from build123d import *

# Parameters (mm, degrees)
BOSS_EXTRUDE1_DEPTH     = 7.62
SKETCH2_W               = 85.677392152
SKETCH2_H               = 16.256
CUT_EXTRUDE1_DEPTH      = 1
CUT_EXTRUDE1_DEPTH_BACK = 8.62
FILLET1_R               = 5.08
SKETCH3_W               = 10.16
SKETCH3_H               = 7.62
CUT_EXTRUDE2_DEPTH      = 8.62
SKETCH4_W               = 25.4
SKETCH4_H               = 10.16
CUT_EXTRUDE3_DEPTH      = 8.62


with BuildPart() as part:
    # Sketch1 → Boss-Extrude1 (new body)
    with BuildSketch(Plane(origin=(0, 0, 0), x_dir=(1, 0, 0), z_dir=(0, 1, 0))):
        with BuildLine():
            Line((-88.9, 0), (-88.9, 76.2))
            ThreePointArc((-88.9, 76.2), (0, 165.1), (88.9, 76.2))
            Line((88.9, 76.2), (88.9, 0))
            ThreePointArc((88.9, 0), (0, -88.9), (-88.9, 0))
        make_face()
    extrude(amount=BOSS_EXTRUDE1_DEPTH)

    # Sketch2 → Cut-Extrude1 (cut, two sides)
    with BuildSketch(Plane(origin=(0, 7.62, 0), x_dir=(1, 0, 0), z_dir=(0, 1, 0))) as cut_extrude1_sk:
        with Locations((0, -58.235236409)):
            Rectangle(SKETCH2_W, SKETCH2_H)
        with Locations((0, 134.435236409)):
            Rectangle(SKETCH2_W, SKETCH2_H)
    extrude(amount=CUT_EXTRUDE1_DEPTH, mode=Mode.SUBTRACT)
    extrude(cut_extrude1_sk.sketch, amount=-CUT_EXTRUDE1_DEPTH_BACK, mode=Mode.SUBTRACT)

    # Fillet1
    fillet1_edges = [part.edges().sort_by_distance(p)[0] for p in [
        (-42.838696076, 3.81, 66.363236409),
        (-42.838696076, 3.81, 50.107236409),
        (42.838696076, 3.81, 50.107236409),
        (42.838696076, 3.81, 66.363236409),
        (-42.838696076, 3.81, -126.307236409),
        (-42.838696076, 3.81, -142.563236409),
        (42.838696076, 3.81, -142.563236409),
        (42.838696076, 3.81, -126.307236409),
    ]]
    fillet(fillet1_edges, radius=FILLET1_R)

    # Sketch3 → Cut-Extrude2 (cut, through all)
    with BuildSketch(Plane(origin=(0, 7.62, 0), x_dir=(1, 0, 0), z_dir=(0, 1, 0))):
        with Locations((10.922, 87.445236409)):
            Rectangle(SKETCH3_W, SKETCH3_H)
        with Locations((-10.922, 87.445236409)):
            Rectangle(SKETCH3_W, SKETCH3_H)
        with Locations((10.922, 120.973236409)):
            Rectangle(SKETCH3_W, SKETCH3_H)
        with Locations((-10.922, 120.973236409)):
            Rectangle(SKETCH3_W, SKETCH3_H)
        with Locations((-10.922, -11.245236409)):
            Rectangle(SKETCH3_W, SKETCH3_H)
        with Locations((10.922, -11.245236409)):
            Rectangle(SKETCH3_W, SKETCH3_H)
        with Locations((-10.922, -44.773236409)):
            Rectangle(SKETCH3_W, SKETCH3_H)
        with Locations((10.922, -44.773236409)):
            Rectangle(SKETCH3_W, SKETCH3_H)
    extrude(amount=-CUT_EXTRUDE2_DEPTH, mode=Mode.SUBTRACT)

    # Sketch4 → Cut-Extrude3 (cut, through all)
    with BuildSketch(Plane(origin=(0, 7.62, 0), x_dir=(1, 0, 0), z_dir=(0, 1, 0))):
        with Locations((0, 67.537940424)):
            Rectangle(SKETCH4_W, SKETCH4_H)
        with Locations((0, 8.662059576)):
            Rectangle(SKETCH4_W, SKETCH4_H)
    extrude(amount=-CUT_EXTRUDE3_DEPTH, mode=Mode.SUBTRACT)


solid = part.part
Read the model definition and answer for the solid it produces. Units are mm, in the model's axes. Coordinates: 2 decimals unless noted, no trailing zeros. Loops run counter-clockwise (first coordinate to the right, second up) from the corner with the lowest first, then second, coordinate; pieces in that order, holes last. Notation, with made-up numbers: (31.25, 49.5) - (89.25, 49.5) arc R30 ccw to (89.25, 75.5) - close; hole circle Ø7 at (34.25, 73.25). An arc over 180 degrees is marked (long way). Answer in a Markdown table with one row per item.
Q1. Given P1, Ø2.5, axis at y = 4.5, z = -85.5, coming from the -X side; P2, Ø4, axis at x = -9, y = 4.5, coming from the +Z side; P3, Ø2.5, axis at y = 2, z = -120.5, coming from the +X side, each flat-ended and moving along its own axis, determine where each tip first touches the part or whether it passes through.
Here are the results:
| item | result |
|---|---|
| P1 | stops at x = -88.53 |
| P2 | stops at z = 88.62 |
| P3 | stops at x = 77.78 |
Q2. The mould has two halves that part along X. Classify faces 1 (the cylindrical face through (-1.95, 3.76, -165.08)), 2 (the flat face through (88.9, 4, -39)), 3 (the flat face through (-11, 4, -124.783)): pulls with the +X half, pulls with the -X half, needs draft (parallel to the pull), parting line crosses it, or undercut.
Here are the results:
| item | result |
|---|---|
| face 1 | parting line crosses it |
| face 2 | pulls with the +X half |
| face 3 | undercut |
Q3. Straight lines are drawn through the part: line 1 along Z through (x, y) = (1, 3.75); line 2 along X through (y, z) = (6.5, 13); line 3 along X through (y, z) = (5.75, -123). For each, find the intervals that lie inside material, in ascending order. Write a range as [from, to].
Here are the results:
| item | result |
|---|---|
| line 1 | z = [-165.09, -142.56], [-126.31, -72.62], [-62.46, -13.74], [-3.58, 50.11], [66.36, 88.89] |
| line 2 | x = [-87.94, -16], [-5.84, 5.84], [16, 87.94] |
| line 3 | x = [-75.58, -16], [-5.84, 5.84], [16, 75.58] |
Q4. Find section C-C on z = 72. Write down the section's boundary in (x, y), plus the area to 3 significant figures.
Here are the results:
| item | result |
|---|---|
| outline | (-52.15, 0) - (52.15, 0) - (52.15, 7.62) - (-52.15, 7.62) - close |
| area | 795 mm^2 |
Q5. Find section B-B on y = 4.75. Count the separate pieces of the cut face and the enclosed holes in it, plus the area to 3 significant figures.
Here are the results:
| item | result |
|---|---|
| separate pieces | 1 |
| enclosed holes | 12 |
| area | 34,500 mm^2 |
Q6. Find section A-A on x = 0. Write down the section's boundary in (y, z).
Here are the results:
| item | result |
|---|---|
| outline | (0, -165.1) - (7.62, -165.1) - (7.62, -142.56) - (0, -142.56) - close; (0, -126.31) - (7.62, -126.31) - (7.62, -72.62) - (0, -72.62) - close; (0, -62.46) - (7.62, -62.46) - (7.62, -13.74) - (0, -13.74) - close; (0, -3.58) - (7.62, -3.58) - (7.62, 50.11) - (0, 50.11) - close; (0, 66.36) - (7.62, 66.36) - (7.62, 88.9) - (0, 88.9) - close |
Q7. Find section D-D on x = 77.5. Write down the section's boundary in (y, z), plus the area to 3 significant figures.
Here are the results:
| item | result |
|---|---|
| outline | (0, -119.75) - (7.62, -119.75) - (7.62, 43.55) - (0, 43.55) - close |
| area | 1,240 mm^2 |
